Verification items for the finished model (mm, model axes). A direction names the side the tool comes from. Coordinates: 2 decimals unless noted, no trailing zeros. Write each loop counter-clockwise with the first axis right and the second up, starting at its lowest first coordinate (ties: lowest second). Pieces come first, ordered by that corner, then holes. Notation, with made-up numbers: (-8.5, 81) -> (0.5, 81) arc R19 ccw to (0.5, 108) -> close; hole circle Ø5 at (86, 17.25). An arc over 180 degrees is marked (long way). Answer in a Markdown table with one row per item.
```python
from build123d import *

# Parameters (mm, degrees)
BOSS_EXTRUDE1_DEPTH     = 15
BOSS_EXTRUDE2_DEPTH     = 10
SKETCH3_R               = 3.25
CUT_EXTRUDE1_DEPTH      = 9
CUT_EXTRUDE2_START      = -7
SKETCH4_R               = 6
CUT_EXTRUDE2_DEPTH      = 7
CHAMFER1_START          = 3
CHAMFER1_2_DEPTH        = 7
CHAMFER1_3_OUTLINE_R    = 12
CHAMFER1_3_OUTLINE_R_2  = 6
CHAMFER1_3_DEPTH        = 7
CHAMFER2_SIZE           = 5
CHAMFER2_SIZE2          = 3
SKETCH5_W               = 22
SKETCH5_H               = 32.792874394
CUT_EXTRUDE3_DEPTH      = 12
FILLET1_R               = 10
FILLET2_R               = 10
BOSS_EXTRUDE3_START     = 3
BOSS_EXTRUDE3_DEPTH     = 3
SKETCH7_W               = 60
SKETCH7_H               = 2
BOSS_EXTRUDE4_DEPTH     = 69
SKETCH8_W               = 60
SKETCH8_H               = 92.343979927
CUT_EXTRUDE4_DEPTH      = 416.45813754
BOSS_EXTRUDE5_START     = 69
BOSS_EXTRUDE5_DEPTH     = 69
CUT_EXTRUDE5_DEPTH      = 396.831589728
CUT_EXTRUDE5_DEPTH_BACK = 396.831589728


with BuildPart() as part:
    # Sketch1 → Boss-Extrude1 (new body)
    with BuildSketch(Plane(origin=(0, 0, 0), x_dir=(1, 0, 0), z_dir=(0, 1, 0))):
        with BuildLine():
            Line((-30, -408.070415552), (30, -408.070415552))
            Line((30, -408.070415552), (30, -372.350901436))
            ThreePointArc((30, -372.350901436), (0, -375.726435625), (-30, -372.350901436))
            Line((-30, -372.350901436), (-30, -408.070415552))
        make_face()
        with BuildLine():
            Line((-21, -395.210658494), (-21, -385.210658494))
            ThreePointArc((-21, -385.210658494), (-23, -383.210658494), (-25, -385.210658494))
            Line((-25, -385.210658494), (-25, -395.210658494))
            ThreePointArc((-25, -395.210658494), (-23, -397.210658494), (-21, -395.210658494))
        make_face(mode=Mode.SUBTRACT)
        with BuildLine():
            Line((25, -385.210658494), (25, -395.210658494))
            ThreePointArc((25, -395.210658494), (23, -397.210658494), (21, -395.210658494))
            Line((21, -395.210658494), (21, -385.210658494))
            ThreePointArc((21, -385.210658494), (23, -383.210658494), (25, -385.210658494))
        make_face(mode=Mode.SUBTRACT)
    extrude(amount=BOSS_EXTRUDE1_DEPTH)

    # Sketch2 → Boss-Extrude2 (add)
    with BuildSketch(Plane(origin=(0, 0, 0), x_dir=(1, 0, 0), z_dir=(0, 1, 0))):
        with BuildLine():
            Line((30, -372.350901436), (19.377517729, -330.775495649))
            ThreePointArc((19.377517729, -330.775495649), (0, -315.726435625), (-19.377517729, -330.775495649))
            Line((-19.377517729, -330.775495649), (-30, -372.350901436))
            ThreePointArc((-30, -372.350901436), (0, -375.726435625), (30, -372.350901436))
        make_face()
    extrude(amount=BOSS_EXTRUDE2_DEPTH)

    # Sketch3 → Cut-Extrude1 (cut)
    with BuildSketch(Plane(origin=(0, 10, 0), x_dir=(1, 0, 0), z_dir=(0, 1, 0))):
        with Locations(Location((0, -335.726435625, 0), (0, 0, 270))):
            Circle(SKETCH3_R)
    extrude(amount=-CUT_EXTRUDE1_DEPTH, mode=Mode.SUBTRACT)

    # Sketch4 → Cut-Extrude2 (cut)
    with BuildSketch(Plane(origin=(0, 10, 0), x_dir=(1, 0, 0), z_dir=(0, 1, 0)).offset(CUT_EXTRUDE2_START)):
        with BuildLine():
            Line((30, -372.350901436), (19.377517729, -330.775495649))
            ThreePointArc((19.377517729, -330.775495649), (0, -315.726435625), (-19.377517729, -330.775495649))
            Line((-19.377517729, -330.775495649), (-30, -372.350901436))
            ThreePointArc((-30, -372.350901436), (0, -375.726435625), (30, -372.350901436))
        make_face()
        with Locations(Location((0, -335.726435625, 0), (0, 0, 270))):
            Circle(SKETCH4_R, mode=Mode.SUBTRACT)
    extrude(amount=CUT_EXTRUDE2_DEPTH, mode=Mode.SUBTRACT)

    # Chamfer1: read off the stored shape, not the designer's step
    # Chamfer1 outline → Chamfer1 (revolve)
    with BuildSketch(Plane.XY.offset(335.726435625)):
        Polygon((26, 3), (12, 10), (12, 3), align=None)
    revolve(axis=Axis((0, 0, 335.726435625), (0, 1, 0)))

    # Chamfer1 2 outline → Chamfer1 2 (cut)
    with BuildSketch(Plane(origin=(0, 0, 0), x_dir=(1, 0, 0), z_dir=(0, 1, 0)).offset(CHAMFER1_START)):
        with BuildLine():
            ThreePointArc((-19.377517729, -330.775495649), (0, -315.726435625), (19.377517729, -330.775495649))
            Line((19.377517729, -330.775495649), (24.033863727, -349))
            Line((24.033863727, -349), (27, -349))
            Line((27, -349), (27, -308))
            Line((27, -308), (-27, -308))
            Line((-27, -308), (-27, -349))
            Line((-27, -349), (-24.033863727, -349))
            Line((-24.033863727, -349), (-19.377517729, -330.775495649))
        make_face()
    extrude(amount=CHAMFER1_2_DEPTH, mode=Mode.SUBTRACT)

    # Chamfer1 3 outline → Chamfer1 3 (add)
    with BuildSketch(Plane(origin=(0, 0, 0), x_dir=(1, 0, 0), z_dir=(0, 1, 0)).offset(CHAMFER1_START)):
        with Locations((0, -335.726435625)):
            Circle(CHAMFER1_3_OUTLINE_R)
        with Locations((0, -335.726435625)):
            Circle(CHAMFER1_3_OUTLINE_R_2, mode=Mode.SUBTRACT)
    extrude(amount=CHAMFER1_3_DEPTH)

    # Chamfer2
    chamfer2_edges = [part.edges().sort_by_distance(p)[0] for p in [
        (0, 10, 332.476435625),
    ]]
    chamfer2_side = [part.faces().sort_by_distance(p)[0] for p in [
        (-11.660588745, 10, 335.726435625),
    ]]
    chamfer(chamfer2_edges, length=CHAMFER2_SIZE, length2=CHAMFER2_SIZE2, reference=chamfer2_side[0])

    # Sketch5 → Cut-Extrude3 (cut)
    with BuildSketch(Plane(origin=(0, 15, 0), x_dir=(1, 0, 0), z_dir=(0, 1, 0))):
        with Locations((0, -391.673978355)):
            Rectangle(SKETCH5_W, SKETCH5_H)
    extrude(amount=-CUT_EXTRUDE3_DEPTH, mode=Mode.SUBTRACT)

    # Fillet1
    fillet1_edges = [part.edges().sort_by_distance(p)[0] for p in [
        (-11, 9, 375.277541158),
        (11, 9, 375.277541158),
    ]]
    fillet(fillet1_edges, radius=FILLET1_R)

    # Fillet2
    fillet2_edges = [part.edges().sort_by_distance(p)[0] for p in [
        (30, 7.5, 408.070415552),
        (-30, 7.5, 408.070415552),
    ]]
    fillet(fillet2_edges, radius=FILLET2_R)

    # Sketch6 → Boss-Extrude3 (add)
    with BuildSketch(Plane.XZ.offset(BOSS_EXTRUDE3_START)):
        with BuildLine():
            Line((-30, 388.070415552), (30, 388.070415552))
            Line((30, 388.070415552), (30, 372.350901436))
            Line((30, 372.350901436), (19.377517729, 330.775495649))
            ThreePointArc((19.377517729, 330.775495649), (0, 315.726435625), (-19.377517729, 330.775495649))
            Line((-19.377517729, 330.775495649), (-30, 372.350901436))
            Line((-30, 372.350901436), (-30, 388.070415552))
        make_face()
    extrude(amount=-BOSS_EXTRUDE3_DEPTH)

    # Sketch7 → Boss-Extrude4 (add)
    with BuildSketch(Plane.XZ.offset(3)):
        with Locations((0, 387.070415552)):
            Rectangle(SKETCH7_W, SKETCH7_H)
    extrude(amount=BOSS_EXTRUDE4_DEPTH)

    # Sketch8 → Cut-Extrude4 (cut, through all)
    with BuildSketch(Plane(origin=(0, 0, 0), x_dir=(1, 0, 0), z_dir=(0, 1, 0))):
        with Locations((0, -361.898425589)):
            Rectangle(SKETCH8_W, SKETCH8_H)
    extrude(amount=CUT_EXTRUDE4_DEPTH, mode=Mode.SUBTRACT)

    # Sketch9 → Boss-Extrude5 (add)
    with BuildSketch(Plane.XZ.offset(3).offset(BOSS_EXTRUDE5_START)):
        with BuildLine():
            Line((-2.5, 386.070415552), (2.5, 386.070415552))
            Line((2.5, 386.070415552), (2.5, 315.883300792))
            ThreePointArc((2.5, 315.883300792), (0, 315.726435625), (-2.5, 315.883300792))
            Line((-2.5, 315.883300792), (-2.5, 386.070415552))
        make_face()
        with BuildLine():
            Line((14.377517729, 386.070415552), (19.377517729, 386.070415552))
            Line((19.377517729, 386.070415552), (19.377517729, 330.775495649))
            ThreePointArc((19.377517729, 330.775495649), (17.460939697, 325.973713704), (14.377517729, 321.823666695))
            Line((14.377517729, 321.823666695), (14.377517729, 386.070415552))
        make_face()
        with BuildLine():
            Line((-19.377517729, 386.070415552), (-19.377517729, 330.775495649))
            ThreePointArc((-19.377517729, 330.775495649), (-17.460939697, 325.973713704), (-14.377517729, 321.823666695))
            Line((-14.377517729, 321.823666695), (-14.377517729, 386.070415552))
            Line((-14.377517729, 386.070415552), (-19.377517729, 386.070415552))
        make_face()
    extrude(amount=-BOSS_EXTRUDE5_DEPTH)

    # Sketch10 → Cut-Extrude5 (cut, two sides: drawn at the far end of the back side and taken through both)
    with BuildSketch(Plane(origin=(0, 0, 0), x_dir=(0, 0, -1), z_dir=(1, 0, 0)).offset(-CUT_EXTRUDE5_DEPTH_BACK)):
        Polygon((-386.070415552, -72), (-315.726435625, -72), (-315.726435625, -3), align=None)
    extrude(amount=CUT_EXTRUDE5_DEPTH + CUT_EXTRUDE5_DEPTH_BACK, mode=Mode.SUBTRACT)


solid = part.part
```
1. Go/stop test with flat-tipped pins: pin 1 (3 mm diameter, centred on x = 25, y = -43.5, fed in from -Z); pin 2 (16.5 mm diameter, centred on y = -48.5, z = 370.5, fed in from -X); pin 3 (20.5 mm diameter, centred on y = -52, z = 362.5, fed in from +X). Record where each tip stops, or that it passes through.
Findings below:
| item | result |
|---|---|
| pin 1 | stops at z = 386.07 |
| pin 2 | stops at x = -19.38 |
| pin 3 | stops at x = 19.38 |
2. Release check for a two-part mould opening along X. For faces 1 (the face through (24, -3, 365)), 2 (the face through (-8, -3, 351)), 3 (the face through (-24.614, -1.521, 351.272)) record: released by +X, released by -X, zero draft, split by the parting line, or undercut.
Findings below:
| item | result |
|---|---|
| face 1 | zero draft |
| face 2 | undercut |
| face 3 | released by -X |
3. Access from +Z, -Z, +X, -X, +Y, -Y to the whole of each face (thin tool, end or side, straight path). Record for faces 4 (the face through (-14.378, -30, 361)), 5 (the face through (25, -37, 386.07)), 6 (the face through (-23, -3, 365)), 7 (the face through (-0.04, -37.02, 350.41)).
Findings below:
| item | result |
|---|---|
| face 4 | -Z, -Y |
| face 5 | -Z, +X, -Y |
| face 6 | -Z, -X, -Y |
| face 7 | -Z, +X, -X, -Y |
4. Sectioned sample at D-D, the plane y = -51. Record the cut outline in (x, z).
Findings below:
| item | result |
|---|---|
| outline | (-30, 386.07) -> (-19.38, 386.07) -> (-19.38, 364.66) -> (-14.38, 364.66) -> (-14.38, 386.07) -> (-2.5, 386.07) -> (-2.5, 364.66) -> (2.5, 364.66) -> (2.5, 386.07) -> (14.38, 386.07) -> (14.38, 364.66) -> (19.38, 364.66) -> (19.38, 386.07) -> (30, 386.07) -> (30, 388.07) -> (-30, 388.07) -> close |
5. Sectioned sample at B-B, the plane z = 329. Record the cut outline in (x, y).
Findings below:
| item | result |
|---|---|
| outline | (-18.83, -16.02) -> (-14.38, -16.02) -> (-14.38, -3) -> (-2.5, -3) -> (-2.5, -16.02) -> (2.5, -16.02) -> (2.5, -3) -> (14.38, -3) -> (14.38, -16.02) -> (18.83, -16.02) -> (18.83, 0) -> (-18.83, 0) -> close |
6. Sectioned sample at A-A, the plane y = -39. Record the cut outline in (x, z), and give its area (3 significant figures).
Findings below:
| item | result |
|---|---|
| outline | (-30, 386.07) -> (-19.38, 386.07) -> (-19.38, 352.43) -> (-14.38, 352.43) -> (-14.38, 386.07) -> (-2.5, 386.07) -> (-2.5, 352.43) -> (2.5, 352.43) -> (2.5, 386.07) -> (14.38, 386.07) -> (14.38, 352.43) -> (19.38, 352.43) -> (19.38, 386.07) -> (30, 386.07) -> (30, 388.07) -> (-30, 388.07) -> close |
| area | 625 mm² |
7. Sectioned sample at C-C, the plane x = -24. Record the cut outline in (y, z).
Findings below:
| item | result |
|---|---|
| outline | (-72, 386.07) -> (-3, 386.07) -> (-3, 348.87) -> (0, 348.87) -> (0, 388.07) -> (-72, 388.07) -> close |
8. Material ranges on probe 1 along X at (y, z) = (-28.5, 384); probe 2 along Y at (x, z) = (-22, 378); probe 3 along Z at (x, y) = (-27, -16), recorded low to high. Write a range as from..to.
Findings below:
| item | result |
|---|---|
| probe 1 | x = -19.38..-14.38, -2.5..2.5, 14.38..19.38 |
| probe 2 | y = -3..0 |
| probe 3 | z = 386.07..388.07 |
